The model under review builds one solid part; all positions refer to its coordinate system, in mm. A direction names the side the tool comes from. Round coordinates to 2 decimals unless told otherwise and drop trailing zeros. Loops run counter-clockwise (first coordinate to the right, second up) from the corner with the lowest first, then second, coordinate; pieces in that order, holes last. Notation, with made-up numbers: (48, -35) -> (88, -35) arc R13 cw to (88, -11) -> close; hole circle Ø11 at (75, 66.5). An arc over 180 degrees is marked (long way). Use a Markdown table: item, result. Add a question column.
1) Wall thickness on probe 1 along X at (y, z) = (8.75, 4); probe 2 along X at (y, z) = (22.5, 2.5); probe 3 along Z at (x, y) = (46.5, 9): over which ranges is each line inside the solid? List them lowest first.
2) Consider section B-B on x = 52.5. Give the boundary of the cut face in (y, z), plus the area to 3 significant figures.
3) Mouldability with a two-part tool opening along Y and no side actions: class faces 1 (the flat face through (38, 0, 10)), 2 (the cylindrical face through (37.2, 18.7, 30.7)), 3 (the flat face through (37, 13, 8.055)) as released by +Y, released by -Y, zero draft, split by the parting line, or undercut.
4) Insertion check: pin 1 (5 mm diameter, centred on x = 53.5, z = 23.5, fed in from -Y); pin 2 (8 mm diameter, centred on y = 19, z = 25.5, fed in from +X); pin 3 (5 mm diameter, centred on x = 22, y = 5, fed in from -Z); pin 4 (13.5 mm diameter, centred on x = 6.5, y = 16, fed in from +Z). Each pin has a flat end and moves straight along its axis. Give the tip position at first contact, or say it passes through.
5) Consider section D-D on y = 13.5. Give the boundary of the cut face in (x, z).
6) Consider section A-A on z = 23.5. Give the boundary of the cut face in (x, y).
7) Consider section C-C on y = 5.5. Give the boundary of the cut face in (x, z).
8) For faces 4 (the flat face through (50, 10, 16.329)), 5 (the flat face through (16.873, 16, 16)), 6 (the flat face through (37, 9, 34.871)), 7 (the flat face through (58.021, 17, 12)), 8 (the flat face through (25, 8, 16.329)), list the 3-axis set-ups (+Z, -Z, +X, -X, +Y, -Y) from which the entire face can be reached by the end or side of a thin tool; tool diameter is ignored.
from build123d import *

# Parameters (mm, degrees)
F1_DEPTH = 25.4
F2_R     = 2.841654
F2_R_2   = 2.530663
F2_R_3   = 3.386715
F2_R_4   = 2.667783
F3_DEPTH = 25.4
F4_R     = 2.244401
F5_DEPTH = 41.148
F6_W     = 8.585986
F6_H     = 17.454494
F7_DEPTH = 18.542


with BuildPart() as f1:
    # F0 (on Front) → F1 (new body)
    with BuildSketch(Plane.XZ):
        Polygon((0, 8.055429), (0, 0), (25.799144, 0), (25.799144, 8.055429), (48.876859, 8.055429), (48.876859, 0), (75.438, 0), (75.438, 8.055429), (58.02086, 8.055429), (58.02086, 16.328571), (16.872857, 16.328571), (16.872857, 8.055429), align=None)
    extrude(amount=-F1_DEPTH)

    # F2 (on face) → F3 (cut)
    with BuildSketch(Plane(origin=(0, 0, 0), x_dir=(1, 0, 0), z_dir=(0, 0, -1))):
        with Locations((12.32334, -6.5187)):
            Circle(F2_R)
        with Locations((11.617891, -17.25835)):
            Circle(F2_R_2)
        with Locations((61.239045, -8.03216)):
            Circle(F2_R_3)
        with Locations((61.239045, -18.230911)):
            Circle(F2_R_4)
    extrude(amount=-F3_DEPTH, mode=Mode.SUBTRACT)

    # F4 (on face) → F5 (join)
    with BuildSketch(Plane(origin=(16.872857, 0, 0), x_dir=(0, -1, 0), z_dir=(-1, 0, 0))):
        with BuildLine():
            Line((-25.4, 31.604629), (-25.4, 16.328571))
            Line((-25.4, 16.328571), (-16.109549, 16.328571))
            Line((-16.109549, 16.328571), (-16.109549, 31.604629))
            ThreePointArc((-16.109549, 31.604629), (-20.754774, 36.249855), (-25.4, 31.604629))
        make_face()
        with Locations((-20.754774, 31.604629)):
            Circle(F4_R, mode=Mode.SUBTRACT)
    extrude(amount=-F5_DEPTH)

    # F6 (on face) → F7 (join)
    with BuildSketch(Plane.XY.offset(16.328571)):
        with Locations((37.301889, 8.727247)):
            Rectangle(F6_W, F6_H)
    extrude(amount=F7_DEPTH)


solid = f1.part
Result set:
| question | item | result |
|---|---|---|
| 1 | probe 1 | 0 to 10.56, 14.08 to 25.8, 48.88 to 57.93, 64.55 to 75.44 |
| 1 | probe 2 | 0 to 25.8, 48.88 to 75.44 |
| 1 | probe 3 | 8.06 to 16.33 |
| 2 | outline | (0, 0) -> (25.4, 0) -> (25.4, 31.6) arc R4.65 ccw to (16.11, 31.6) -> (16.11, 16.33) -> (0, 16.33) -> close; hole circle Ø4.49 at (20.75, 31.6) |
| 2 | area | 575 mm2 |
| 3 | face 1 | released by -Y |
| 3 | face 2 | undercut |
| 3 | face 3 | zero draft |
| 4 | pin 1 | y = 16.11 |
| 4 | pin 2 | x = 58.02 |
| 4 | pin 3 | z = 0 |
| 4 | pin 4 | z = 8.06 |
| 5 | outline | (0, 0) -> (25.8, 0) -> (25.8, 8.06) -> (48.88, 8.06) -> (48.88, 0) -> (75.44, 0) -> (75.44, 8.06) -> (58.02, 8.06) -> (58.02, 16.33) -> (41.59, 16.33) -> (41.59, 34.87) -> (33.01, 34.87) -> (33.01, 16.33) -> (16.87, 16.33) -> (16.87, 8.06) -> (0, 8.06) -> close |
| 6 | outline | (16.87, 16.11) -> (33.01, 16.11) -> (33.01, 0) -> (41.59, 0) -> (41.59, 16.11) -> (58.02, 16.11) -> (58.02, 25.4) -> (16.87, 25.4) -> close |
| 7 | outline | (0, 0) -> (9.67, 0) -> (9.67, 8.06) -> (0, 8.06) -> close; (14.98, 0) -> (25.8, 0) -> (25.8, 8.06) -> (48.88, 8.06) -> (48.88, 0) -> (58.99, 0) -> (58.99, 8.06) -> (58.02, 8.06) -> (58.02, 16.33) -> (41.59, 16.33) -> (41.59, 34.87) -> (33.01, 34.87) -> (33.01, 16.33) -> (16.87, 16.33) -> (16.87, 8.06) -> (14.98, 8.06) -> close; (63.49, 0) -> (75.44, 0) -> (75.44, 8.06) -> (63.49, 8.06) -> close |
| 8 | face 4 | +Z, +X, -Y |
| 8 | face 5 | +Z, -X, +Y, -Y |
| 8 | face 6 | +Z, +X, -X, -Y |
| 8 | face 7 | +Z, +X, +Y, -Y |
| 8 | face 8 | +Z, -X, -Y |
